Geometry: final body of the model. Coordinates: model frame, mm. Coordinates: 2 decimals unless noted, no trailing zeros. Write each loop counter-clockwise with the first axis right and the second up, starting at its lowest first coordinate (ties: lowest second). Pieces come first, ordered by that corner, then holes. Notation, with made-up numbers: (-31, -11) -> (-10, -11) arc R8 ccw to (-10, -1) -> close; hole circle Ø11 at (43.5, 86.25). An arc over 180 degrees is marked (long way). One line per item, written item: value.
```python
from build123d import *

# Parameters (mm, degrees)
SKETCH_1_R          = 1.59
EXTRUDE_1_DEPTH     = 1.57
CUT_EXTRUDE_1_DEPTH = 84.57


with BuildPart() as part:
    # 草图1 → 凸台-拉伸1 (new body)
    with BuildSketch(Plane(origin=(0, 0, 0), x_dir=(1, 0, 0), z_dir=(0, 1, 0))):
        with BuildLine():
            ThreePointArc((50.6, -0.95), (49.65, 0), (48.7, -0.95))
            Line((48.7, -0.95), (48.7, -9.35))
            Line((48.7, -9.35), (37.5, -9.35))
            Line((37.5, -9.35), (37.5, 3.4))
            Line((37.5, 3.4), (33.85, 3.4))
            Line((33.85, 3.4), (33.85, -4.85))
            Line((33.85, -4.85), (25.85, -4.85))
            Line((25.85, -4.85), (25.85, 3.4))
            Line((25.85, 3.4), (7.5, 3.4))
            Line((7.5, 3.4), (7.5, -4.85))
            Line((7.5, -4.85), (-7.5, -4.85))
            Line((-7.5, -4.85), (-7.5, 4.85))
            Line((-7.5, 4.85), (-7.5, 48.85))
            Line((-7.5, 48.85), (-7.5, 59.55))
            Line((-7.5, 59.55), (160.15, 59.55))
            Line((160.15, 59.55), (160.15, 3.4))
            Line((160.15, 3.4), (121.8, 3.4))
            Line((121.8, 3.4), (121.8, -9.35))
            Line((121.8, -9.35), (50.6, -9.35))
            Line((50.6, -9.35), (50.6, -0.95))
        make_face()
        with Locations(Location((0, 53.9, 0), (0, 0, 270))):
            Circle(SKETCH_1_R, mode=Mode.SUBTRACT)
        with Locations(Location((0, 0, 0), (0, 0, 270))):
            Circle(SKETCH_1_R, mode=Mode.SUBTRACT)
    extrude(amount=EXTRUDE_1_DEPTH)

    # 草图2 → 切除-拉伸1 (cut)
    with BuildSketch(Plane(origin=(121.8, 0, 0), x_dir=(0, 0, -1), z_dir=(1, 0, 0))):
        Polygon((-9.35, 1.096838695), (-8.05, 1.57), (-9.35, 1.57), align=None)
        Polygon((-8.05, 0), (-9.35, 0.473161305), (-9.35, 0), align=None)
    extrude(amount=-CUT_EXTRUDE_1_DEPTH, mode=Mode.SUBTRACT)


solid = part.part
```
(1) Section A-A (x = 0). Return the cut outline in (y, z).
Responses:
outline: (0, -59.55) -> (1.57, -59.55) -> (1.57, -55.49) -> (0, -55.49) -> close; (0, -52.31) -> (1.57, -52.31) -> (1.57, -1.59) -> (0, -1.59) -> close; (0, 1.59) -> (1.57, 1.59) -> (1.57, 4.85) -> (0, 4.85) -> close
(2) Section B-B (z = -53.9). Return the cut outline in (x, y).
Responses:
outline: (-7.5, 0) -> (-1.59, 0) -> (-1.59, 1.57) -> (-7.5, 1.57) -> close; (1.59, 0) -> (160.15, 0) -> (160.15, 1.57) -> (1.59, 1.57) -> close
(3) First-contact query: pin 1 (0.8 mm diameter, centred on x = 31.5, y = 1, fed in from +Z); pin 2 (0.8 mm diameter, centred on x = 15, y = 1, fed in from +Z); pin 3 (0.8 mm diameter, centred on y = 1, z = 0.5, fed in from +X). Flat tips, straight axial feed; report the tip coordinate or a pass-through.
Responses:
pin 1: stops at z = 4.85
pin 2: stops at z = -3.4
pin 3: stops at x = 121.8
(4) Section C-C (x = 23). Return the cut outline in (y, z), then the cut area to 3 significant figures.
Responses:
outline: (0, -59.55) -> (1.57, -59.55) -> (1.57, -3.4) -> (0, -3.4) -> close
area: 88.2 mm2
(5) Line query: line 1 (X direction, y = 0.5, z = 6.5); line 2 (X direction, y = 1, z = 0.5); line 3 (X direction, y = 0.7, z = -53.9). Output: solid intervals per line, ascending. Write a range as [from, to].
Responses:
line 1: x = [37.5, 48.7], [50.6, 121.8]
line 2: x = [-7.5, -1.51], [1.51, 7.5], [25.85, 33.85], [37.5, 48.81], [50.49, 121.8]
line 3: x = [-7.5, -1.59], [1.59, 160.15]
(6) Pull-direction query (Z, two-part tool) for faces 1 (the cylindrical face through (0.07, 0.77, -55.49)), 2 (the flat face through (77, 0, -26)); classes: released by +Z, released by -Z, zero draft, split by the parting line, or undercut.
Responses:
face 1: undercut
face 2: zero draft
